Study the drawing (mm; zero at the part's minimum x, y, z) and answer. A direction names the side the tool comes from. Coordinates: 2 decimals unless noted, no trailing zeros. Loops run counter-clockwise (first coordinate to the right, second up) from the corner with the lowest first, then second, coordinate; pieces in that order, holes last. Notation, with made-up numbers: (-26.5, -7.75) -> (16.5, -7.75) arc R17 ccw to (16.5, 3.25) -> close; hole circle Ø8 at (58.25, 62). An arc over 180 degrees is marked (long way). Answer in a Markdown table with one row per item.
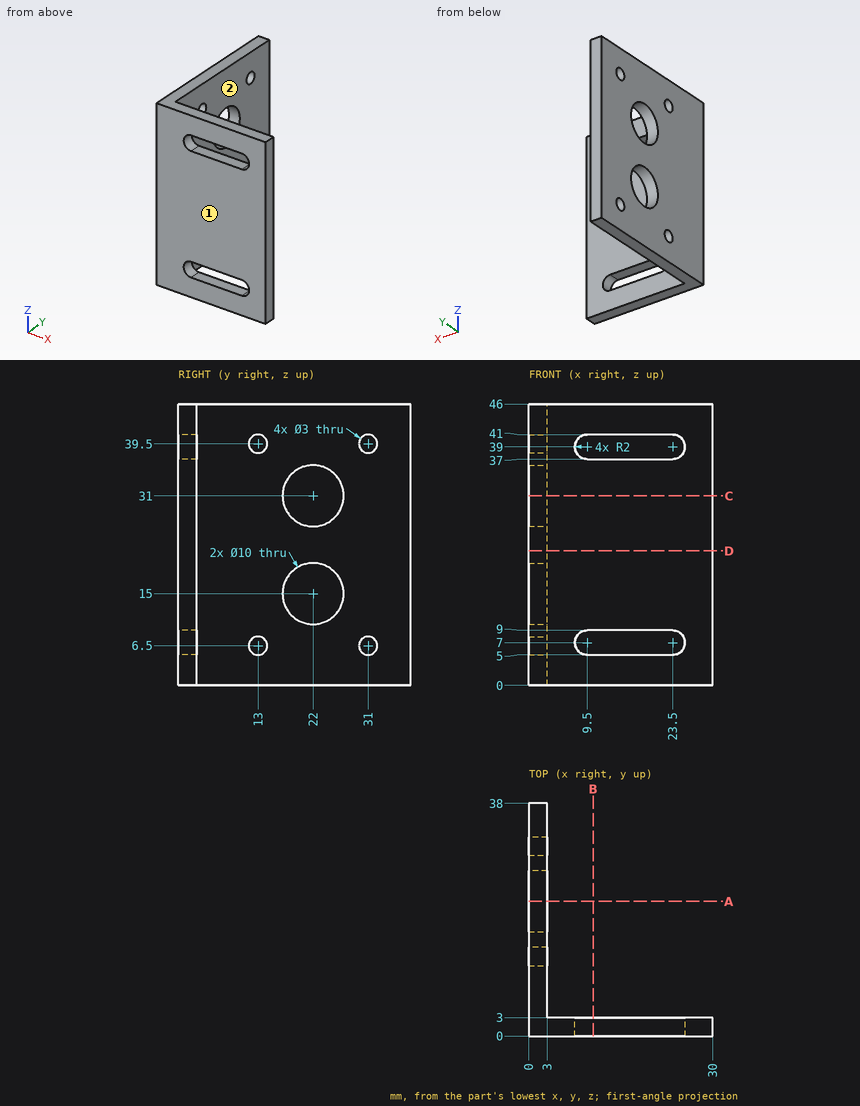
1. Given pin 1 Ø4 at (y, z) = (13, 39.5) entering from -X; pin 2 Ø8 at (x, z) = (10, 14.5) entering from +Y; pin 3 Ø8 at (y, z) = (22, 15) entering from +X; pin 4 Ø4 at (y, z) = (13, 6.5) entering from +X, each flat-ended and moving along its own axis, determine where each tip first touches the part or whether it passes through.
A:
| item | result |
|---|---|
| pin 1 | stops at x = 0 |
| pin 2 | stops at y = 3 |
| pin 3 | passes through |
| pin 4 | stops at x = 3 |
2. A cutting plane is placed at C-C on z = 31. Give the vertices of the cut face in (x, y).
A:
| item | result |
|---|---|
| outline | (0, 0) -> (30, 0) -> (30, 3) -> (3, 3) -> (3, 17) -> (0, 17) -> close; (0, 27) -> (3, 27) -> (3, 38) -> (0, 38) -> close |
3. Find the intervals of material crossed by probe 1 along Z at (x, y) = (0.65, 22); probe 2 along Z at (x, y) = (1.8, 31); probe 3 along X at (y, z) = (8, 20), in increasing order.
A:
| item | result |
|---|---|
| probe 1 | z = 0 to 10, 20 to 26, 36 to 46 |
| probe 2 | z = 0 to 5, 8 to 38, 41 to 46 |
| probe 3 | x = 0 to 3 |
4. A cutting plane is placed at D-D on z = 22. Give the vertices of the cut face in (x, y), and give its area (3 significant figures).
A:
| item | result |
|---|---|
| outline | (0, 0) -> (30, 0) -> (30, 3) -> (3, 3) -> (3, 38) -> (0, 38) -> close |
| area | 195 mm2 |
5. A cutting plane is placed at B-B on x = 10.5. Give the vertices of the cut face in (y, z).
A:
| item | result |
|---|---|
| outline | (0, 0) -> (3, 0) -> (3, 5) -> (0, 5) -> close; (0, 9) -> (3, 9) -> (3, 37) -> (0, 37) -> close; (0, 41) -> (3, 41) -> (3, 46) -> (0, 46) -> close |
6. A tool of negligible diameter and unlimited length cuts with its end or side. For the marked faces 1 and 2, from which of +Z, -Z, +X, -X, +Y, -Y can it reach the whole face along a straight path? Write none if from no direction.
A:
| item | result |
|---|---|
| face 1 | +Z, -Z, +X, -X, -Y |
| face 2 | +Z, -Z, +X, +Y |
7. A cutting plane is placed at A-A on y = 22. Give the vertices of the cut face in (x, z).
A:
| item | result |
|---|---|
| outline | (0, 0) -> (3, 0) -> (3, 10) -> (0, 10) -> close; (0, 20) -> (3, 20) -> (3, 26) -> (0, 26) -> close; (0, 36) -> (3, 36) -> (3, 46) -> (0, 46) -> close |
